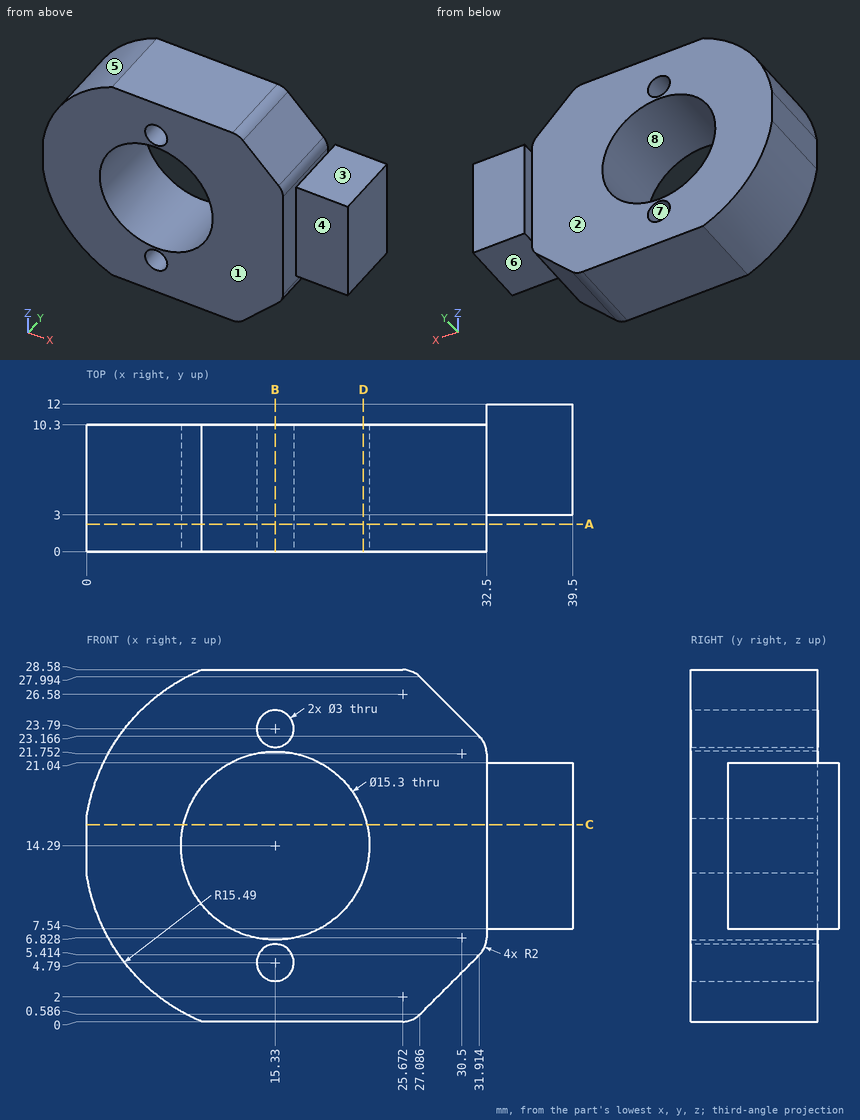
Can you work these out from the drawing? Everything is in mm from the part's minimum corner. A direction names the side the tool comes from. Round coordinates to 2 decimals unless told otherwise and drop trailing zeros. Loops run counter-clockwise (first coordinate to the right, second up) from the corner with the lowest first, then second, coordinate; pieces in that order, holes last.
1. If we section it at A-A on y = 2.25: Count the separate pieces of the cut face and the enclosed holes in it, plus the area to 3 significant figures.
Answer list:
separate pieces: 1
enclosed holes: 3
area: 623 mm2
2. If we section it at D-D on x = 22.5: Write out the boundary of the cut face in (y, z).
Answer list:
outline: (0, 0) - (10.3, 0) - (10.3, 11.62) - (0, 11.62) - close; (0, 16.96) - (10.3, 16.96) - (10.3, 28.58) - (0, 28.58) - close
3. We'd pull the mould along Z, two halves only. Please class the marked faces 5, 6, 7 and 8: +Z half, -Z half, draft (parallel to the pull), parting line (faces both ways), or undercut.
Answer list:
face 5: +Z half
face 6: -Z half
face 7: undercut
face 8: undercut
4. For P1, Ø14.5, axis at x = 23.5, z = 18, coming from the +Y side; P2, Ø1.9, axis at y = 11.5, z = 14.5, coming from the -X side; P3, Ø1.5, axis at y = 8.5, z = 25.5, coming from the +X side, each with a flat end and sliding along its axis, tell me the tip position at first contact or that it passes through.
Answer list:
P1: stops at y = 10.3
P2: stops at x = 32.5
P3: stops at x = 30.33
5. If we section it at B-B on x = 15.33: Write out the boundary of the cut face in (y, z).
Answer list:
outline: (0, 0) - (10.3, 0) - (10.3, 3.29) - (0, 3.29) - close; (0, 6.29) - (10.3, 6.29) - (10.3, 6.64) - (0, 6.64) - close; (0, 21.94) - (10.3, 21.94) - (10.3, 22.29) - (0, 22.29) - close; (0, 25.29) - (10.3, 25.29) - (10.3, 28.58) - (0, 28.58) - close
6. Which directions (+Z, -Z, +X, -X, +Y, -Y) give clear straight access to the entire face, cutting with the end or side of a thin tool? Please do the marked faces 1, 2, 3 and 4.
Answer list:
face 1: +Z, -Z, +X, -X, -Y
face 2: +Z, -Z, -X, +Y
face 3: +Z, +X, +Y, -Y
face 4: +Z, -Z, +X, -Y
7. If we section it at C-C on z = 16: Write out the boundary of the cut face in (x, y).
Answer list:
outline: (0, 0) - (7.87, 0) - (7.87, 10.3) - (0, 10.3) - close; (22.79, 0) - (32.5, 0) - (32.5, 3) - (39.5, 3) - (39.5, 12) - (32.5, 12) - (32.5, 10.3) - (22.79, 10.3) - close
8. If I drill on line 1 along X through (y, z) = (4.5, 14.29); line 2 along Y through (x, z) = (19, 21.75); line 3 along X through (y, z) = (2.5, 14.29), over which ranges is the centre line in solid material (lowest first)?
Answer list:
line 1: x = 0 to 7.68, 22.98 to 39.5
line 2: y = 0 to 10.3
line 3: x = 0 to 7.68, 22.98 to 32.5
